Here's how the part is built. I have some questions about the finished solid (model axes, mm). Face numbers are marked on the shaded views. A direction names the side the tool comes from. Coordinates: 2 decimals unless noted, no trailing zeros. Order: outer loops, then holes, each group sorted by start corner. A loop starts at its lowest first (then second) coordinate and runs counter-clockwise, first axis right, second up. Notation, with made-up numbers: (67, 35) - (81, 35) arc R22 cw to (81, 49) - close; hole circle Ø6 at (64.25, -1). An arc over 180 degrees is marked (long way). Answer as CSV lines item,"result". Start each with the question number.
Item 1: We'd pull the mould along X, two halves only. Please class the marked faces 1, 2, 3 and 4: pulls with the +X half, pulls with the -X half, needs draft (parallel to the pull), parting line crosses it, or undercut.
Item 2: Imagine slicing it at D-D on x = 15.5. List the corners of the cut face in (y, z) for me, and give its area (3 significant figures).
Item 3: On a 3-axis mill with a long thin cutter (end or side, diameter ignored), from which of +Z, -Z, +X, -X, +Y, -Y can I reach the whole of each face in a straight line? I mean the marked faces 5, 6 and 7. Say none if no direction works.
Item 4: Imagine slicing it at A-A on z = -19. List the corners of the cut face in (x, y) for me, and give its area (3 significant figures).
Item 5: I'm going to push flat-ended pins straight in: pin 1 (3 mm diameter, centred on x = 12, z = -3, fed in from +Y); pin 2 (2 mm diameter, centred on y = 3, z = -29, fed in from -X); pin 3 (2.5 mm diameter, centred on y = 3, z = -25.5, fed in from -X); pin 4 (2 mm diameter, centred on x = -6.5, z = 1.5, fed in from -Y). Where does each tip first touch, or does it pass through?
Item 6: Imagine slicing it at C-C on y = 9. List the corners of the cut face in (x, z) for me.
Item 7: I need wall thicknesses on line 1 (Z direction, x = 16, y = 2.75); line 2 (Y direction, x = -15, z = -25); line 3 (X direction, y = 4.75, z = 0). Which ranges of each line are inside material? Lowest first, please.
from build123d import *

# Parameters (mm, degrees)
BRACKET_DEPTH       = 11.5
BOSS_EXTRUDE1_START = -3
BOSS_EXTRUDE1_DEPTH = 3
CUT_EXTRUDE1_START  = -3
CUT_EXTRUDE1_DEPTH  = 2
CUT_EXTRUDE2_START  = -2.5
SKETCH15_4_W        = 5
SKETCH15_4_H        = 5
CUT_EXTRUDE2_DEPTH  = 2.5


with BuildPart() as part:
    # Sketch9 → Bracket (new body)
    with BuildSketch(Plane(origin=(0, 0, 0), x_dir=(1, 0, 0), z_dir=(0, 1, 0))):
        with BuildLine():
            Line((5.15, -5), (4.65, -5))
            Line((4.65, -5), (3.35, -5))
            Line((3.35, -5), (3.35, -7))
            Line((3.35, -7), (6.4, -7))
            ThreePointArc((6.4, -7), (6.930330086, -6.780330086), (7.15, -6.25))
            Line((7.15, -6.25), (7.15, -5))
            Line((7.15, -5), (7.15, -3.25))
            ThreePointArc((7.15, -3.25), (7.369669914, -2.719669914), (7.9, -2.5))
            Line((7.9, -2.5), (21.4, -2.5))
            ThreePointArc((21.4, -2.5), (21.930330086, -2.280330086), (22.15, -1.75))
            Line((22.15, -1.75), (22.15, 24.75))
            ThreePointArc((22.15, 24.75), (21.930330086, 25.280330086), (21.4, 25.5))
            Line((21.4, 25.5), (7.9, 25.5))
            ThreePointArc((7.9, 25.5), (7.369669914, 25.719669914), (7.15, 26.25))
            Line((7.15, 26.25), (7.15, 28))
            Line((7.15, 28), (7.15, 29.75))
            ThreePointArc((7.15, 29.75), (6.930330086, 30.280330086), (6.4, 30.5))
            Line((6.4, 30.5), (5.15, 30.5))
            Line((5.15, 30.5), (3.35, 30.5))
            Line((3.35, 30.5), (3.35, 28.5))
            Line((3.35, 28.5), (5.15, 28.5))
            Line((5.15, 28.5), (5.15, 28))
            Line((5.15, 28), (5.15, 23.5))
            Line((5.15, 23.5), (20.15, 23.5))
            Line((20.15, 23.5), (20.15, -0.5))
            Line((20.15, -0.5), (5.15, -0.5))
            Line((5.15, -0.5), (5.15, -5))
        make_face()
    extrude(amount=BRACKET_DEPTH)

    # Sketch12 → Boss-Extrude1 (add)
    with BuildSketch(Plane(origin=(0, 0, 0), x_dir=(1, 0, 0), z_dir=(0, 1, 0)).offset(BOSS_EXTRUDE1_START)):
        with BuildLine():
            Line((3.134136634, -6.799408153), (-15.169112008, 10.208954707))
            ThreePointArc((-15.169112008, 10.208954707), (-17.445237733, 24.907700028), (-3.6745965, 30.529381479))
            ThreePointArc((-3.6745965, 30.529381479), (-3.571695801, 30.507381696), (-3.466728879, 30.5))
            Line((-3.466728879, 30.5), (6.4, 30.5))
            ThreePointArc((6.4, 30.5), (6.930330086, 30.280330086), (7.15, 29.75))
            Line((7.15, 29.75), (7.15, 26.25))
            ThreePointArc((7.15, 26.25), (7.369669914, 25.719669914), (7.9, 25.5))
            Line((7.9, 25.5), (21.4, 25.5))
            ThreePointArc((21.4, 25.5), (21.930330086, 25.280330086), (22.15, 24.75))
            Line((22.15, 24.75), (22.15, -1.75))
            ThreePointArc((22.15, -1.75), (21.930330086, -2.280330086), (21.4, -2.5))
            Line((21.4, -2.5), (7.9, -2.5))
            ThreePointArc((7.9, -2.5), (7.369669914, -2.719669914), (7.15, -3.25))
            Line((7.15, -3.25), (7.15, -6.25))
            ThreePointArc((7.15, -6.25), (6.930330086, -6.780330086), (6.4, -7))
            Line((6.4, -7), (3.644676233, -7))
            ThreePointArc((3.644676233, -7), (3.370410043, -6.948053048), (3.134136634, -6.799408153))
        make_face()
    extrude(amount=BOSS_EXTRUDE1_DEPTH)

    # Sketch15 → Cut-Extrude1 (cut)
    with BuildSketch(Plane(origin=(0, 0, 0), x_dir=(1, 0, 0), z_dir=(0, 1, 0)).offset(CUT_EXTRUDE1_START)):
        with BuildLine():
            Line((-9.279054633, 12.306278316), (-8.999521572, 7.000514852))
            ThreePointArc((-8.999521572, 7.000514852), (-6.999521572, 5.000514852), (-4.999521572, 7.000514852))
            Line((-4.999521572, 7.000514852), (-4.720515244, 12.306424778))
            ThreePointArc((-4.720515244, 12.306424778), (-1.999839357, 14.000160648), (-0.306278316, 16.720945367))
            Line((-0.306278316, 16.720945367), (4.999485148, 17.000478428))
            ThreePointArc((4.999485148, 17.000478428), (6.999485148, 19.000478428), (4.999485148, 21.000478428))
            Line((4.999485148, 21.000478428), (-0.306424778, 21.279484756))
            ThreePointArc((-0.306424778, 21.279484756), (-2.000160648, 24.000160643), (-4.720945367, 25.693721684))
            Line((-4.720945367, 25.693721684), (-5.000478428, 30.999485148))
            ThreePointArc((-5.000478428, 30.999485148), (-7.000478428, 32.999485148), (-9.000478428, 30.999485148))
            Line((-9.000478428, 30.999485148), (-9.279484756, 25.693575222))
            ThreePointArc((-9.279484756, 25.693575222), (-12.000160643, 23.999839352), (-13.693721684, 21.279054633))
            Line((-13.693721684, 21.279054633), (-18.999485148, 20.999521572))
            ThreePointArc((-18.999485148, 20.999521572), (-20.999485148, 18.999521572), (-18.999485148, 16.999521572))
            Line((-18.999485148, 16.999521572), (-13.693575222, 16.720515244))
            ThreePointArc((-13.693575222, 16.720515244), (-11.999839352, 13.999839357), (-9.279054633, 12.306278316))
        make_face()
    extrude(amount=CUT_EXTRUDE1_DEPTH, mode=Mode.SUBTRACT)

    # Sketch15<4> → Cut-Extrude2 (cut)
    with BuildSketch(Plane(origin=(0, 0, 0), x_dir=(1, 0, 0), z_dir=(0, 1, 0)).offset(CUT_EXTRUDE2_START)):
        with BuildLine():
            Line((-13.693721684, 21.279054633), (-9.5, 21.5))
            Line((-9.5, 21.5), (-9.279484756, 25.693575222))
            ThreePointArc((-9.279484756, 25.693575222), (-12.000160643, 23.999839352), (-13.693721684, 21.279054633))
        make_face()
        with BuildLine():
            Line((-9.5, 21.5), (-7.000099677, 21.5))
            Line((-7.000099677, 21.5), (-7.000281928, 26.071067806))
            ThreePointArc((-7.000281928, 26.071067806), (-8.155404343, 25.976033314), (-9.279484756, 25.693575222))
            Line((-9.279484756, 25.693575222), (-9.5, 21.5))
        make_face()
        with BuildLine():
            Line((-7.000099677, 21.5), (-4.5, 21.5))
            Line((-4.5, 21.5), (-4.720945367, 25.693721684))
            ThreePointArc((-4.720945367, 25.693721684), (-5.845097933, 25.976116485), (-7.000281928, 26.071067806))
            Line((-7.000281928, 26.071067806), (-7.000099677, 21.5))
        make_face()
        with BuildLine():
            Line((-4.720945367, 25.693721684), (-4.5, 21.5))
            Line((-4.5, 21.5), (-0.306424778, 21.279484756))
            ThreePointArc((-0.306424778, 21.279484756), (-2.000160648, 24.000160643), (-4.720945367, 25.693721684))
        make_face()
        with BuildLine():
            Line((-0.306278316, 16.720945367), (-4.5, 16.5))
            Line((-4.5, 16.5), (-4.720515244, 12.306424778))
            ThreePointArc((-4.720515244, 12.306424778), (-1.999839357, 14.000160648), (-0.306278316, 16.720945367))
        make_face()
        with BuildLine():
            Line((-0.306424778, 21.279484756), (-4.5, 21.5))
            Line((-4.5, 21.5), (-4.5, 16.5))
            Line((-4.5, 16.5), (-0.306278316, 16.720945367))
            ThreePointArc((-0.306278316, 16.720945367), (-0.023906539, 17.844958862), (0.071067812, 19))
            ThreePointArc((0.071067812, 19), (-0.023943654, 20.155265273), (-0.306424778, 21.279484756))
        make_face()
        with Locations((-7, 19)):
            Rectangle(SKETCH15_4_W, SKETCH15_4_H)
        with BuildLine():
            Line((-4.720515244, 12.306424778), (-4.5, 16.5))
            Line((-4.5, 16.5), (-9.5, 16.5))
            Line((-9.5, 16.5), (-9.279054633, 12.306278316))
            ThreePointArc((-9.279054633, 12.306278316), (-6.999772812, 11.928932192), (-4.720515244, 12.306424778))
        make_face()
        with BuildLine():
            Line((-9.5, 16.5), (-9.5, 21.5))
            Line((-9.5, 21.5), (-13.693721684, 21.279054633))
            ThreePointArc((-13.693721684, 21.279054633), (-14.071067808, 18.999772812), (-13.693575222, 16.720515244))
            Line((-13.693575222, 16.720515244), (-9.5, 16.5))
        make_face()
        with BuildLine():
            Line((-9.279054633, 12.306278316), (-9.5, 16.5))
            Line((-9.5, 16.5), (-13.693575222, 16.720515244))
            ThreePointArc((-13.693575222, 16.720515244), (-11.999839352, 13.999839357), (-9.279054633, 12.306278316))
        make_face()
    extrude(amount=CUT_EXTRUDE2_DEPTH, mode=Mode.SUBTRACT)


solid = part.part
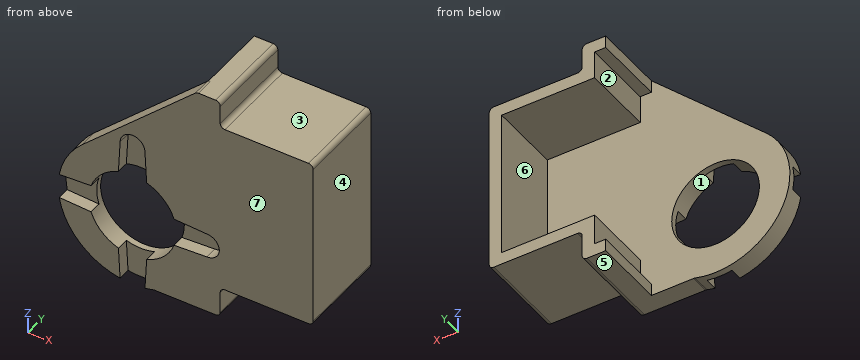
Responses:
1,face 1,"undercut"
1,face 2,"pulls with the -X half"
1,face 3,"needs draft"
1,face 4,"pulls with the +X half"
2,outline,"(-3, -25.5) - (11.5, -25.5) - (11.5, -23.5) - (0, -23.5) - (0, 0.5) - (11.5, 0.5) - (11.5, 2.5) - (-3, 2.5) - close"
2,area,"130 mm^2"
3,face 5,"-Z, +X, +Y, -Y"
3,face 6,"-X, +Y"
3,face 7,"+Z, -Z, +X, -X, -Y"
4,outline,"(-19, -1) - (-14.07, -1) - (-14.07, 0) - (-19, 0) - close; (0.07, -1) - (7, -1) - (7, -3) - (22.15, -3) - (22.15, 11.5) - (20.15, 11.5) - (20.15, 0) - (0.07, 0) - close"
4,area,"80.3 mm^2"
5,pin 1,"stops at y = 0"
5,pin 2,"stops at x = 3.35"
5,pin 3,"stops at x = 5.15"
5,pin 4,"passes through"
6,outline,"(3.35, -30.5) - (6.4, -30.5) arc R0.75 ccw to (7.15, -29.75) - (7.15, -26.25) arc R0.75 cw to (7.9, -25.5) - (21.4, -25.5) arc R0.75 ccw to (22.15, -24.75) - (22.15, 1.75) arc R0.75 ccw to (21.4, 2.5) - (7.9, 2.5) arc R0.75 cw to (7.15, 3.25) - (7.15, 6.25) arc R0.75 ccw to (6.4, 7) - (3.35, 7) - (3.35, 5) - (5.15, 5) - (5.15, 0.5) - (20.15, 0.5) - (20.15, -23.5) - (5.15, -23.5) - (5.15, -28.5) - (3.35, -28.5) - close"
7,line 1,"z = -25.5 to -23.5, 0.5 to 2.5"
7,line 2,"y = -3 to 0"
7,line 3,"x = 20.15 to 22.15"
